from build123d import *

# Parameters (mm, degrees)
SKETCH_2_W          = 94.005
SKETCH_2_H          = 52.73
EXTRUDE_1_DEPTH     = 4
FILLET_1_R          = 2
M2_5X0_45_1_D       = 2.05
CUT_EXTRUDE_1_DEPTH = 1
SKETCH_8_W          = 10
SKETCH_8_H          = 12
SKETCH_8_W_2        = 12
SKETCH_8_H_2        = 10
CUT_EXTRUDE_2_DEPTH = 2
FILLET_2_R          = 1


with BuildPart() as part:
    # 草图2 → 凸台-拉伸1 (new body)
    with BuildSketch(Plane(origin=(0, 0, 0), x_dir=(1, 0, 0), z_dir=(0, 1, 0))):
        with Locations((150.1775, -79.375)):
            Rectangle(SKETCH_2_W, SKETCH_2_H)
    extrude(amount=-EXTRUDE_1_DEPTH)

    # 圆角1
    fillet_1_edges = [part.edges().sort_by_distance(p)[0] for p in [
        (197.18, -2, 53.01),
        (197.18, -2, 105.74),
        (103.175, -2, 105.74),
        (103.175, -2, 53.01),
    ]]
    fillet(fillet_1_edges, radius=FILLET_1_R)

    # M2.5x0.45 螺纹孔1 (through all)
    with Locations(Plane(origin=(109.855, 0, 58.42), x_dir=(0, 0, 1), z_dir=(0, 1, 0))):
        with Locations((0, 0), (41.91, 0), (34.29, 31.75), (22.932, 26.615), (22.932, 10.215), (6.532, 10.215), (6.532, 26.615), (6.532, 37.52), (22.932, 37.52), (22.932, 53.92), (6.532, 53.92), (0, 78.74), (41.91, 72.39), (0, 31.75)):
            Hole(M2_5X0_45_1_D / 2)

    # 草图7 → 切除-拉伸1 (cut)
    with BuildSketch(Plane(origin=(0, 0, 0), x_dir=(1, 0, 0), z_dir=(0, 1, 0))):
        with BuildLine():
            Line((118.42, -62.302), (138.12, -62.302))
            ThreePointArc((138.12, -62.302), (138.827106781, -62.594893219), (139.12, -63.302))
            Line((139.12, -63.302), (139.12, -83.002))
            ThreePointArc((139.12, -83.002), (138.827106781, -83.709106781), (138.12, -84.002))
            Line((138.12, -84.002), (118.42, -84.002))
            ThreePointArc((118.42, -84.002), (117.712893219, -83.709106781), (117.42, -83.002))
            Line((117.42, -83.002), (117.42, -63.302))
            ThreePointArc((117.42, -63.302), (117.712893219, -62.594893219), (118.42, -62.302))
        make_face()
        with BuildLine():
            Line((145.725, -62.302), (165.425, -62.302))
            ThreePointArc((165.425, -62.302), (166.132106781, -62.594893219), (166.425, -63.302))
            Line((166.425, -63.302), (166.425, -83.002))
            ThreePointArc((166.425, -83.002), (166.132106781, -83.709106781), (165.425, -84.002))
            Line((165.425, -84.002), (145.725, -84.002))
            ThreePointArc((145.725, -84.002), (145.017893219, -83.709106781), (144.725, -83.002))
            Line((144.725, -83.002), (144.725, -63.302))
            ThreePointArc((144.725, -63.302), (145.017893219, -62.594893219), (145.725, -62.302))
        make_face()
    extrude(amount=-CUT_EXTRUDE_1_DEPTH, mode=Mode.SUBTRACT)

    # 草图8 → 切除-拉伸2 (cut)
    with BuildSketch(Plane(origin=(0, 0, 0), x_dir=(1, 0, 0), z_dir=(0, 1, 0))):
        with Locations((108.175, -68.752)):
            Rectangle(SKETCH_8_W, SKETCH_8_H)
        with Locations((192.18, -68.758)):
            Rectangle(SKETCH_8_W, SKETCH_8_H)
        with Locations((154.178, -100.74)):
            Rectangle(SKETCH_8_W_2, SKETCH_8_H_2)
    extrude(amount=-CUT_EXTRUDE_2_DEPTH, mode=Mode.SUBTRACT)

    # 圆角2
    fillet_2_edges = [part.edges().sort_by_distance(p)[0] for p in [
        (113.175, -1, 62.752),
        (113.175, -1, 74.752),
        (187.18, -1, 74.758),
        (187.18, -1, 62.758),
        (148.178, -1, 95.74),
        (160.178, -1, 95.74),
    ]]
    fillet(fillet_2_edges, radius=FILLET_2_R)


solid = part.part
Work out the finished part from the listing and answer in its coordinate system (mm). A direction names the side the tool comes from. Round coordinates to 2 decimals unless told otherwise and drop trailing zeros. Order: outer loops, then holes, each group sorted by start corner. A loop starts at its lowest first (then second) coordinate and runs counter-clockwise, first axis right, second up. Notation, with made-up numbers: M 11,-19 L 56,-19 A11 cw 56,-15 Z; hole C -30,-3 d10. An arc over 180 degrees is marked long. One line per item, written item: value.
Q1. Find section A-A on z = 100.33. Write down the section's boundary in (x, y) (3 decimals), then the cut area to 3 significant figures.
Derived:
outline: M 103.175,-4 L 108.83,-4 L 108.83,0 L 103.175,0 Z; M 110.88,-4 L 181.22,-4 L 181.22,0 L 160.178,0 L 160.178,-2 L 148.178,-2 L 148.178,0 L 110.88,0 Z; M 183.27,-4 L 197.18,-4 L 197.18,0 L 183.27,0 Z
area: 336 mm²
Q2. Find section C-C on z = 58.42. Write down the section's boundary in (x, y) (3 decimals).
Derived:
outline: M 103.175,-4 L 108.83,-4 L 108.83,0 L 103.175,0 Z; M 110.88,-4 L 140.58,-4 L 140.58,0 L 110.88,0 Z; M 142.63,-4 L 187.57,-4 L 187.57,0 L 142.63,0 Z; M 189.62,-4 L 197.18,-4 L 197.18,0 L 189.62,0 Z
Q3. For faces 1 (the face through (154, -1, 95.74)), 2 (the face through (108, -2, 69)), 3 (the face through (192, -2, 69)), determine the directions among +Z, -Z, +X, -X, +Y, -Y from which every point of the face is accessible in a straight line to the end or side of a thin tool.
Derived:
face 1: +Z, +Y
face 2: -X, +Y
face 3: +X, +Y
Q4. Straight lines are drawn through the part: line 1 (X direction, y = -0.9, z = 58.42) (3 decimals); line 2 (X direction, y = -2.1, z = 92.71) (3 decimals); line 3 (Z direction, x = 120.5, y = -0.95). For each, find the intervals that lie inside material, in ascending order.
Derived:
line 1: 103.175 to 108.83, 110.88 to 140.58, 142.63 to 187.57, 189.62 to 197.18
line 2: 103.175 to 140.58, 142.63 to 197.18
line 3: 53.01 to 62.3, 84 to 105.74
Q5. Flat-ended cylindrical pins translate along their axes: pin 1 (10 mm diameter, centred on x = 167.5, z = 60.5, fed in from +Y); pin 2 (1.1 mm diameter, centred on y = -0.5, z = 74, fed in from +X); pin 3 (0.5 mm diameter, centred on y = -0.5, z = 70, fed in from -X) (3 decimals). Find the tip coordinate at first contact, or state that the pin passes through.
Derived:
pin 1: y = 0
pin 2: x = 187.57
pin 3: x = 113.175
Q6. Determine the mould class of faces 4 (the face through (187.18, -1, 69)), 5 (the face through (136.778, -2.521, 63.974)), 6 (the face through (150, -2, 53.01)) for opening direction X: released by +X, released by -X, zero draft, split by the parting line, or undercut.
Derived:
face 4: released by +X
face 5: undercut
face 6: zero draft
Q7. Find section D-D on z = 92.71. Write down the section's boundary in (x, y) (3 decimals), then the cut area to 3 significant figures.
Derived:
outline: M 103.175,-4 L 140.58,-4 L 140.58,0 L 103.175,0 Z; M 142.63,-4 L 197.18,-4 L 197.18,0 L 142.63,0 Z
area: 368 mm²
Q8. Find section B-B on x = 120.07. Write down the section's boundary in (y, z).
Derived:
outline: M -4,53.01 L 0,53.01 L 0,62.3 L -1,62.3 L -1,63.93 L -4,63.93 Z; M -4,65.98 L -1,65.98 L -1,80.33 L -4,80.33 Z; M -4,82.38 L -1,82.38 L -1,84 L 0,84 L 0,105.74 L -4,105.74 Z
